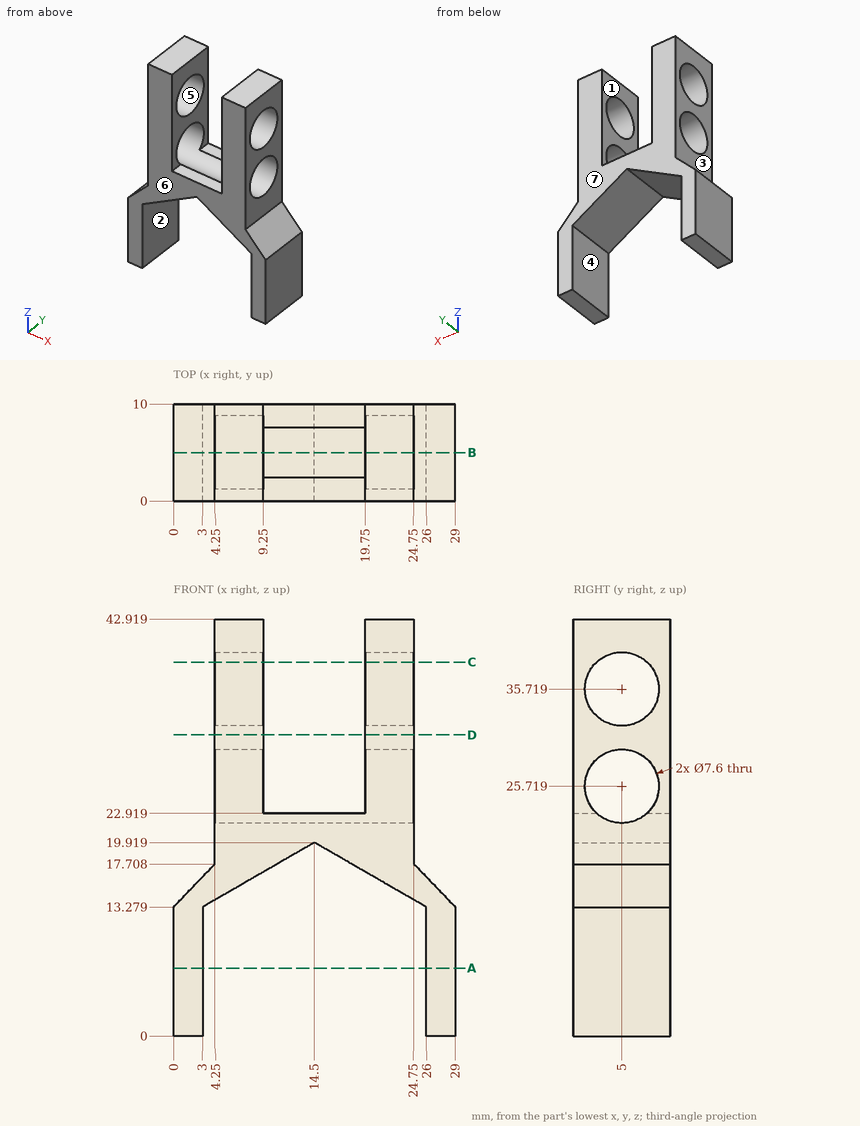
Answer from the drawing. Dimensions are ordinates in mm from the lowest x, y and z of the part. A direction names the side the tool comes from. Coordinates: 2 decimals unless noted, no trailing zeros. Write each loop counter-clockwise with the first axis right and the second up, starting at its lowest first coordinate (ties: lowest second). Pieces come first, ordered by that corner, then holes. Notation, with made-up numbers: M 3,-20.75 L 37,-20.75 A31 cw 37,3.25 Z; hole C -16,32.5 d5. An arc over 180 degrees is marked long. Write item = value, one per line.
1. Determine the mould class of the marked faces 4, 5, 6 and 7 for opening direction Y: released by +Y, released by -Y, zero draft, split by the parting line, or undercut.
Solution:
face_4 = zero draft
face_5 = undercut
face_6 = released by -Y
face_7 = released by +Y
2. For the marked faces 1, 2 and 3, determine the directions among +Z, -Z, +X, -X, +Y, -Y from which every point of the face is accessible in a straight line to the end or side of a thin tool.
Solution:
face_1 = +Z, +Y, -Y
face_2 = -Z, +Y, -Y
face_3 = +Z, -X, +Y, -Y
3. Flat-ended cylindrical pins translate along their axes: pin 1 (1 mm diameter, centred on y = 3, z = 31.5, fed in from -X); pin 2 (1.2 mm diameter, centred on x = 16, y = 1.5, fed in from +Z); pin 3 (5 mm diameter, centred on y = 3.5, z = 24.5, fed in from +X). Find the tip coordinate at first contact, or state that the pin passes through.
Solution:
pin_1 = 4.25
pin_2 = 22.92
pin_3 = 24.75
4. The part is cut by section B-B (y = 5). State how many separate pieces and enclosed holes the cut face has, then the cut area to 3 significant figures.
Solution:
separate_pieces = 5
enclosed_holes = 0
area = 257 mm2
5. The part is cut by section D-D (z = 31). Determine the outline of the cut face in (x, y), then the cut area to 3 significant figures.
Solution:
outline = M 4.25,0 L 9.25,0 L 9.25,10 L 4.25,10 Z; M 19.75,0 L 24.75,0 L 24.75,10 L 19.75,10 Z
area = 100 mm2
6. The part is cut by section A-A (z = 7). Determine the outline of the cut face in (x, y).
Solution:
outline = M 0,0 L 3,0 L 3,10 L 0,10 Z; M 26,0 L 29,0 L 29,10 L 26,10 Z
7. Straight lines are drawn through the part: line 1 (X direction, y = 7.75, z = 11.5); line 2 (X direction, y = 8, z = 31.5); line 3 (Z direction, x = 7, y = 4) (1 decimal). For each, find the intervals that lie inside material, in ascending order. Write a range as from..to.
Solution:
line_1 = 0..3, 26..29
line_2 = 4.25..9.25, 19.75..24.75
line_3 = 15.6..22.1, 29.4..32.1, 39.4..42.9
8. The part is cut by section C-C (z = 38.5). Determine the outline of the cut face in (x, y).
Solution:
outline = M 4.25,0 L 9.25,0 L 9.25,2.41 L 4.25,2.41 Z; M 4.25,7.59 L 9.25,7.59 L 9.25,10 L 4.25,10 Z; M 19.75,0 L 24.75,0 L 24.75,2.41 L 19.75,2.41 Z; M 19.75,7.59 L 24.75,7.59 L 24.75,10 L 19.75,10 Z
